Read the model definition and answer for the solid it produces. Units are mm, in the model's axes. A direction names the side the tool comes from. Round coordinates to 2 decimals unless told otherwise and drop trailing zeros. Write each loop counter-clockwise with the first axis right and the second up, starting at its lowest first coordinate (ties: lowest second). Pieces come first, ordered by that corner, then holes.
from build123d import *

# Parameters (mm, degrees)
SKETCH2_W           = 9.8
SKETCH2_H           = 15
BOSS_EXTRUDE1_DEPTH = 0.6
SKETCH3_W           = 9.8
SKETCH3_H           = 13
BOSS_EXTRUDE2_DEPTH = 3.15
CUT_EXTRUDE1_DEPTH  = 0.254


with BuildPart() as part:
    # Sketch2 → Boss-Extrude1 (new body)
    with BuildSketch(Plane.XY):
        Rectangle(SKETCH2_W, SKETCH2_H)
    extrude(amount=BOSS_EXTRUDE1_DEPTH)

    # Sketch3 → Boss-Extrude2 (add)
    with BuildSketch(Plane.XY.offset(0.6)):
        Rectangle(SKETCH3_W, SKETCH3_H)
    extrude(amount=BOSS_EXTRUDE2_DEPTH)

    # Sketch8 → Cut-Extrude1 (cut)
    with BuildSketch(Plane.XY.offset(3.75)):
        with BuildLine():
            Line((-2.723886994, 0.579326575), (-2.150500712, 3.831161775))
            ThreePointArc((-2.150500712, 3.831161775), (-1.767978563, 4.099006667), (-1.500133672, 3.716484519))
            Line((-1.500133672, 3.716484519), (-2.073519954, 0.464649318))
            ThreePointArc((-2.073519954, 0.464649318), (-2.456042103, 0.196804426), (-2.723886994, 0.579326575))
        make_face()
        with BuildLine():
            Line((3.499725709, 3.820673425), (2.926339427, 0.568838225))
            ThreePointArc((2.926339427, 0.568838225), (2.543817278, 0.300993333), (2.275972387, 0.683515481))
            Line((2.275972387, 0.683515481), (2.849358669, 3.935350682))
            ThreePointArc((2.849358669, 3.935350682), (3.231880818, 4.203195574), (3.499725709, 3.820673425))
        make_face()
        with BuildLine():
            Line((-3.499725709, -3.820673425), (-2.926339427, -0.568838225))
            ThreePointArc((-2.926339427, -0.568838225), (-2.543817278, -0.300993333), (-2.275972387, -0.683515481))
            Line((-2.275972387, -0.683515481), (-2.849358669, -3.935350682))
            ThreePointArc((-2.849358669, -3.935350682), (-3.231880818, -4.203195574), (-3.499725709, -3.820673425))
        make_face()
        with BuildLine():
            Line((1.500133672, -3.716484519), (2.073519954, -0.464649318))
            ThreePointArc((2.073519954, -0.464649318), (2.456042103, -0.196804426), (2.723886994, -0.579326575))
            Line((2.723886994, -0.579326575), (2.150500712, -3.831161775))
            ThreePointArc((2.150500712, -3.831161775), (1.767978563, -4.099006667), (1.500133672, -3.716484519))
        make_face()
        with BuildLine():
            Line((-2.299838715, -4.0698), (0.748161285, -4.0698))
            ThreePointArc((0.748161285, -4.0698), (1.078361285, -4.4), (0.748161285, -4.7302))
            Line((0.748161285, -4.7302), (-2.299838715, -4.7302))
            ThreePointArc((-2.299838715, -4.7302), (-2.630038715, -4.4), (-2.299838715, -4.0698))
        make_face()
        with BuildLine():
            Line((-1.524, 0.3302), (1.524, 0.3302))
            ThreePointArc((1.524, 0.3302), (1.8542, 0), (1.524, -0.3302))
            Line((1.524, -0.3302), (-1.524, -0.3302))
            ThreePointArc((-1.524, -0.3302), (-1.8542, 0), (-1.524, 0.3302))
        make_face()
        with BuildLine():
            Line((-0.748161285, 4.7302), (2.299838715, 4.7302))
            ThreePointArc((2.299838715, 4.7302), (2.630038715, 4.4), (2.299838715, 4.0698))
            Line((2.299838715, 4.0698), (-0.748161285, 4.0698))
            ThreePointArc((-0.748161285, 4.0698), (-1.078361285, 4.4), (-0.748161285, 4.7302))
        make_face()
    extrude(amount=-CUT_EXTRUDE1_DEPTH, mode=Mode.SUBTRACT)


solid = part.part
Q1. Which of the six approach directions +Z, -Z, +X, -X, +Y, -Y give full straight-line access (tool end or side, diameter ignored) to faces 1 (the flat face through (2, -2, 3.496)), 2 (the flat face through (0, 7, 0.6)), 3 (the flat face through (0, 0, 0)), 4 (the flat face through (0, -7, 0.6))?
Verdict:
face 1: +Z
face 2: +Z, +X, -X, +Y
face 3: -Z, +X, -X, +Y, -Y
face 4: +Z, +X, -X, -Y
Q2. Section C-C (y = -4.5) is taken. Determine the outline of the cut face in (x, z), then the cut area to 3 significant figures.
Verdict:
outline: (-4.9, 0) - (4.9, 0) - (4.9, 3.75) - (1.06, 3.75) - (1.06, 3.5) - (-2.61, 3.5) - (-2.61, 3.75) - (-4.9, 3.75) - close
area: 35.8 mm2
Q3. Section B-B (z = 1.1) is taken. Determine the outline of the cut face in (x, y), then the cut area to 3 significant figures.
Verdict:
outline: (-4.9, -6.5) - (4.9, -6.5) - (4.9, 6.5) - (-4.9, 6.5) - close
area: 127 mm2
Q4. Flat-ended cylindrical pins translate along their axes: pin 1 Ø2 at (x, z) = (2.5, 2) entering from +Y; pin 2 Ø1.6 at (x, z) = (0, 1.5) entering from -Y. Find the tip coordinate at first contact, or state that the pin passes through.
Verdict:
pin 1: stops at y = 6.5
pin 2: stops at y = -6.5
Q5. Section A-A (y = 4.4) is taken. Determine the outline of the cut face in (x, z), then the cut area to 3 significant figures.
Verdict:
outline: (-4.9, 0) - (4.9, 0) - (4.9, 3.75) - (2.63, 3.75) - (2.63, 3.5) - (-1.08, 3.5) - (-1.08, 3.75) - (-4.9, 3.75) - close
area: 35.8 mm2
Q6. Straight lines are drawn through the part: probe 1 along X at (y, z) = (3.75, 3.6); probe 2 along Y at (x, z) = (-0.25, 1.7). For each, find the intervals that lie inside material, in ascending order.
Verdict:
probe 1: x = -4.9 to -2.16, -1.5 to 2.82, 3.49 to 4.9
probe 2: y = -6.5 to 6.5
Q7. Determine the mould class of faces 5 (the flat face through (3, 2, 3.496)), 6 (the flat face through (4.9, 0, 2)), 7 (the flat face through (0, -6.5, 2)) for opening direction X: pulls with the +X half, pulls with the -X half, needs draft (parallel to the pull), parting line crosses it, or undercut.
Verdict:
face 5: undercut
face 6: pulls with the +X half
face 7: needs draft
